Could you check a few things on this model? Use its own coordinates, in mm. A direction names the side the tool comes from. Give positions to 0.01 mm unless a question says otherwise; leave off trailing zeros. One line per item, written item: value. Start each with the question number.
Q1. I want a section at A-A (y = 52). Count the separate pieces of the cut face and the enclosed holes in it, then the cut area to 3 significant figures.
Q2. For faces 1 (the face through (-2, 70.104, -41)), 2 (the face through (98.872, 34.738, 0.709)), 3 (the face through (-1.23, 57.58, 32.92)), which set-ups out of +Z, -Z, +X, -X, +Y, -Y let a thin tool reach every point of the face, with its end or its side?
Q3. If I drill on line 1 (Z direction, x = 5, y = 55); line 2 (Z direction, x = 82.5, y = 60.5); line 3 (Y direction, x = -42, z = -1), over which ranges is the centre line in solid material (lowest first)? Write a range as from..to.
Q4. If we mould it in two halves opening along Z, with no side actions, what happens to faces 4 (the face through (-1, 44.704, 0)), 5 (the face through (-7, 0, -51))? For each: released by +Z, released by -Z, zero draft, split by the parting line, or undercut.
Q5. I'm going to push flat-ended pins straight in: P1, Ø3, axis at x = 45, z = -33, coming from the +Y side; P2, Ø12, axis at x = 54.5, z = -4.5, coming from the -Y side; P3, Ø8, axis at y = 21.5, z = 1, coming from the +X side. Where does each tip first touch, or does it pass through?
```python
from build123d import *

# Parameters (mm, degrees)
SKETCH1_W           = 205.785682804
SKETCH1_H           = 104.534748446
BOSS_EXTRUDE1_DEPTH = 70.104
BOSS_EXTRUDE1_TAPER = 4
SKETCH2_W           = 145.758865666
SKETCH2_H           = 50.974097726
CUT_EXTRUDE1_DEPTH  = 25.4
DRAFT1_ANGLE        = 30
SHELL1_T            = -1.5875


with BuildPart() as part:
    # Sketch1 → Boss-Extrude1 (new body)
    with BuildSketch(Plane(origin=(0, 0, 0), x_dir=(1, 0, 0), z_dir=(0, 1, 0))):
        Rectangle(SKETCH1_W, SKETCH1_H)
    extrude(amount=BOSS_EXTRUDE1_DEPTH, taper=BOSS_EXTRUDE1_TAPER)

    # Sketch2 → Cut-Extrude1 (cut)
    with BuildSketch(Plane(origin=(0, 70.104, 0), x_dir=(1, 0, 0), z_dir=(0, 1, 0))):
        Rectangle(SKETCH2_W, SKETCH2_H)
    extrude(amount=-CUT_EXTRUDE1_DEPTH, mode=Mode.SUBTRACT)

    # Draft1
    draft1_faces = [part.faces().sort_by_distance(p)[0] for p in [
        (0, 57.404, 25.487048863),
        (72.879432833, 57.404, 0),
        (0, 57.404, -25.487048863),
        (-72.879432833, 57.404, 0),
    ]]
    draft(draft1_faces, Plane.ZX.offset(44.704), DRAFT1_ANGLE)

    # Shell1
    shell1_openings = [part.faces().sort_by_distance(p)[0] for p in [
        (0, 0, 0),
    ]]
    offset(amount=SHELL1_T, openings=shell1_openings, kind=Kind.INTERSECTION)


solid = part.part
```
Worked answers:
1. separate pieces: 2
1. enclosed holes: 2
1. area: 1,730 mm²
2. face 1: +Z, -Z, +X, -X, +Y
2. face 2: -Y
2. face 3: +Y
3. line 1: z = -48.42..-46.83, -33.26..-31.43, 31.43..33.26, 46.83..48.42
3. line 2: z = -48.04..-46.45, -36.44..36.44, 46.45..48.04
3. line 3: y = 43.12..44.7
4. face 4: undercut
4. face 5: zero draft
5. P1: stops at y = 60.31
5. P2: stops at y = 43.12
5. P3: stops at x = 101.67
